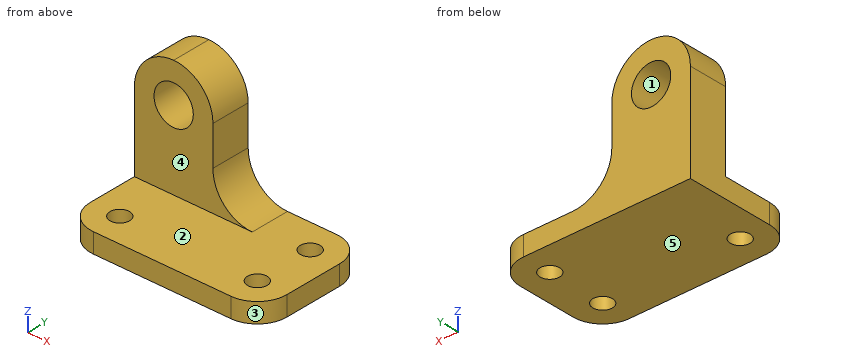
```python
from build123d import *

# Parameters (mm, degrees)
F1_DEPTH  = 38.1
F2_W      = 25.4
F2_H      = 38.1
F3_DEPTH  = 38.101
F4_R      = 6.35
F5_DEPTH  = 12.701
F7_DEPTH  = 12.701
F8_R      = 3.175
F9_DEPTH  = 6.351
F11_DEPTH = 6.351


with BuildPart() as f1:
    # F0 (on Front) → F1 (new body)
    with BuildSketch(Plane.XZ):
        Polygon((-127.4177515995, 134.0467518509), (-165.5177515995, 134.0467518509), (-165.5177515995, 89.5967518509), (-102.0177515995, 89.5967518509), (-102.0177515995, 95.9467518509), (-127.4177515995, 95.9467518509), align=None)
    extrude(amount=F1_DEPTH)

    # F2 (on face) → F3 (cut, through all)
    with BuildSketch(Plane.YZ.offset(-127.4177515995)):
        with Locations((-25.4, 114.9967518509)):
            Rectangle(F2_W, F2_H)
    extrude(amount=-F3_DEPTH, mode=Mode.SUBTRACT)

    # F4 (on face) → F5 (cut, through all)
    with BuildSketch(Plane.XZ.offset(12.7)):
        with Locations((-152.8177515995, 121.3467518509)):
            Circle(F4_R)
        with BuildLine():
            ThreePointArc((-165.5177515995, 121.3467518509), (-161.7980077206, 130.327007972), (-152.8177515995, 134.0467518509))
            Line((-152.8177515995, 134.0467518509), (-165.5177515995, 134.0467518509))
            Line((-165.5177515995, 134.0467518509), (-165.5177515995, 121.3467518509))
        make_face()
    extrude(amount=-F5_DEPTH, mode=Mode.SUBTRACT)

    # F6 (on face) → F7 (cut, through all)
    with BuildSketch(Plane.XZ.offset(12.7)):
        with BuildLine():
            ThreePointArc((-152.8177515995, 134.0467518509), (-143.8630113716, 130.3524515711), (-140.1179560774, 121.4188191659))
            Line((-140.1179560774, 121.4188191659), (-140.1177515995, 108.7188191676))
            ThreePointArc((-140.1177515995, 108.7188191676), (-136.423523409, 99.6919990849), (-127.4177515995, 95.9467518509))
            Line((-127.4177515995, 95.9467518509), (-127.4177515995, 134.0467518509))
            Line((-127.4177515995, 134.0467518509), (-152.8177515995, 134.0467518509))
        make_face()
    extrude(amount=-F7_DEPTH, mode=Mode.SUBTRACT)

    # F8 (on face) → F9 (cut, through all)
    with BuildSketch(Plane.XY.offset(95.9467518509)):
        with Locations((-155.9927515995, -28.575)):
            Circle(F8_R)
        with Locations((-111.5427515995, -28.575)):
            Circle(F8_R)
        with Locations((-111.5427515995, -9.525)):
            Circle(F8_R)
    extrude(amount=-F9_DEPTH, mode=Mode.SUBTRACT)

    # F10 (on face) → F11 (cut, through all)
    with BuildSketch(Plane.XY.offset(95.9467518509)):
        with BuildLine():
            ThreePointArc((-155.9927515995, -38.1), (-162.7279436903, -35.3101920908), (-165.5177515995, -28.575))
            Line((-165.5177515995, -28.575), (-165.5177515995, -38.1))
            Line((-165.5177515995, -38.1), (-155.9927515995, -38.1))
        make_face()
        with BuildLine():
            ThreePointArc((-102.0177515995, -28.575), (-104.8075595087, -35.3101920908), (-111.5427515995, -38.1))
            Line((-111.5427515995, -38.1), (-102.0177515995, -38.1))
            Line((-102.0177515995, -38.1), (-102.0177515995, -28.575))
        make_face()
        with BuildLine():
            Line((-102.0177515995, 0), (-111.5427515995, 0))
            ThreePointArc((-111.5427515995, 0), (-104.8075595087, -2.7898079092), (-102.0177515995, -9.525))
            Line((-102.0177515995, -9.525), (-102.0177515995, 0))
        make_face()
    extrude(amount=-F11_DEPTH, mode=Mode.SUBTRACT)


solid = f1.part
```
Work out the finished part from the listing and answer in its coordinate system (mm). Face numbers are marked on the shaded views. A direction names the side the tool comes from. Give positions to 0.01 mm unless a question says otherwise; leave off trailing zeros. Loops run counter-clockwise (first coordinate to the right, second up) from the corner with the lowest first, then second, coordinate; pieces in that order, holes last. Notation, with made-up numbers: M 79,-14.75 L 99,-14.75 A23 ccw 99,9.25 Z; hole C -11.5,6.25 d5. An arc over 180 degrees is marked long. One line per item, written item: value. Start each with the question number.
1. Find the intervals of material crossed by probe 1 along X at (y, z) = (-29.5, 95); probe 2 along Z at (x, y) = (-143.5, -19.5); probe 3 along X at (y, z) = (-5.5, 118.5), in increasing order.
2. Find section B-B (y = -27.5). Give the vertices of the cut face in (x, z), and give its area (3 significant figures).
3. Find section D-D (y = -3). Give the vertices of the cut face in (x, z).
4. Determine the mould class of the marked faces 1, 2 and 3 for opening direction X: released by +X, released by -X, zero draft, split by the parting line, or undercut.
5. Find section A-A (x = -155). Give the vertices of the cut face in (y, z), and give its area (3 significant figures).
6. Which of the six approach directions +Z, -Z, +X, -X, +Y, -Y give full straight-line access (tool end or side, diameter ignored) to the marked faces 4 and 5?
7. Each of these flat-tipped pins is pushed along its axis until it touches: P1, Ø1.5, axis at x = -151, y = -28, coming from the +Z side; P2, Ø6.5, axis at y = -6.5, z = 112.5, coming from the +X side; P3, Ø1.5, axis at y = -6.5, z = 124, coming from the +X side. Where does it stop, or does it pass through?
8. Find section C-C (z = 120.5). Give the vertices of the cut face in (x, y).
Reported:
1. probe 1: x = -165.47 to -159.03, -152.96 to -114.58, -108.51 to -102.06
1. probe 2: z = 89.6 to 95.95
1. probe 3: x = -165.52 to -158.49, -147.14 to -140.12
2. outline: M -165.52,89.6 L -158.98,89.6 L -158.98,95.95 L -165.52,95.95 Z; M -153.01,89.6 L -114.53,89.6 L -114.53,95.95 L -153.01,95.95 Z; M -108.56,89.6 L -102.02,89.6 L -102.02,95.95 L -108.56,95.95 Z
2. area: 327 mm²
3. outline: M -165.52,89.6 L -104.6,89.6 L -104.6,95.95 L -127.42,95.95 A12.7 cw -140.12,108.72 L -140.12,121.42 A12.7 ccw -165.52,121.35 Z; hole C -152.82,121.35 d12.7
4. face 1: undercut
4. face 2: zero draft
4. face 3: released by +X
5. outline: M -38.1,89.6 L -31.59,89.6 L -31.59,95.95 L -38.1,95.95 Z; M -25.56,89.6 L 0,89.6 L 0,115.38 L -12.7,115.38 L -12.7,95.95 L -25.56,95.95 Z; M -12.7,127.31 L 0,127.31 L 0,133.86 L -12.7,133.86 Z
5. area: 534 mm²
6. face 4: +Z, +X, -X, -Y
6. face 5: -Z, +X, -X, +Y, -Y
7. P1: stops at z = 95.95
7. P2: stops at x = -140.12
7. P3: stops at x = -140.26
8. outline: M -165.52,-12.7 L -159.11,-12.7 L -159.11,0 L -165.52,0 Z; M -146.52,-12.7 L -140.12,-12.7 L -140.12,0 L -146.52,0 Z
